Could you check a few things on this drawing? It's one solid part, dimensions in mm from its lowest x, y, z. A direction names the side the tool comes from. Coordinates: 2 decimals unless noted, no trailing zeros. Write each loop counter-clockwise with the first axis right and the second up, starting at its lowest first coordinate (ties: lowest second). Pieces come first, ordered by that corner, then holes. Notation, with made-up numbers: M 45,5.25 L 72,5.25 A20 cw 72,19.25 Z; hole C -14,36.25 d5. An arc over 180 degrees is marked long. Use a Markdown table: item, result.
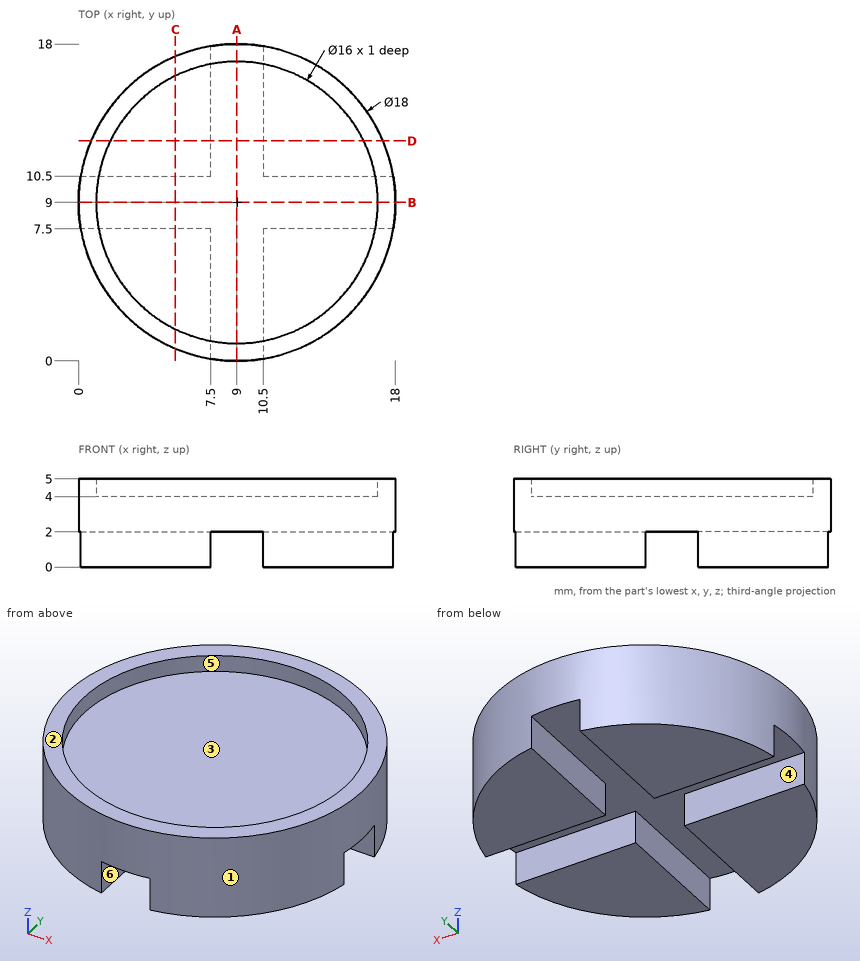
1. Will these pins go through, and if not, where does the flat tip stop? pin 1 Ø2 at (x, z) = (15.5, 1.5) entering from +Y; pin 2 Ø1 at (y, z) = (5.5, 1) entering from +X; pin 3 Ø0.6 at (x, z) = (2.5, 1) entering from -Y.
Answers follow:
| item | result |
|---|---|
| pin 1 | stops at y = 16.12 |
| pin 2 | stops at x = 17.49 |
| pin 3 | stops at y = 2.48 |
2. Suppose I cut it at A-A on x = 9. Write out the boundary of the cut face in (y, z), and give its area (3 significant figures).
Answers follow:
| item | result |
|---|---|
| outline | M 0,2 L 18,2 L 18,5 L 17,5 L 17,4 L 1,4 L 1,5 L 0,5 Z |
| area | 38.0 mm2 |
3. Suppose I cut it at C-C on x = 5.5. Write out the boundary of the cut face in (y, z).
Answers follow:
| item | result |
|---|---|
| outline | M 0.71,0 L 7.5,0 L 7.5,2 L 10.5,2 L 10.5,0 L 17.29,0 L 17.29,5 L 16.19,5 L 16.19,4 L 1.81,4 L 1.81,5 L 0.71,5 Z |
4. Which directions (+Z, -Z, +X, -X, +Y, -Y) give clear straight access to the entire face, cutting with the end or side of a thin tool? Please do the marked faces 4, 5 and 6.
Answers follow:
| item | result |
|---|---|
| face 4 | -Z, +X, -X |
| face 5 | +Z |
| face 6 | -Z, +Y, -Y |
5. We'd pull the mould along X, two halves only. Please class the marked faces 1, 2 and 3: +X half, -X half, draft (parallel to the pull), parting line (faces both ways), or undercut.
Answers follow:
| item | result |
|---|---|
| face 1 | parting line |
| face 2 | draft |
| face 3 | undercut |
6. I need wall thicknesses on probe 1 along Y at (x, z) = (9, 4.5); probe 2 along Z at (x, y) = (10.75, 3.5); probe 3 along Y at (x, z) = (4, 1.7). Which ranges of each line are inside material? Lowest first, please.
Answers follow:
| item | result |
|---|---|
| probe 1 | y = 0 to 1, 17 to 18 |
| probe 2 | z = 0 to 4 |
| probe 3 | y = 1.52 to 7.5, 10.5 to 16.48 |
